Check sheet for the drawn part. Datum: minimum x, y, z corner. Units: mm. A direction names the side the tool comes from. Round coordinates to 2 decimals unless told otherwise and drop trailing zeros. Write each loop counter-clockwise with the first axis right and the second up, starting at its lowest first coordinate (ties: lowest second). Pieces come first, ordered by that corner, then holes. Notation, with made-up numbers: M -33.75,29.5 L -25.75,29.5 A26 cw -25.75,68.5 Z; hole C 55.5,6.5 d8. An arc over 180 degrees is marked long. One line per item, written item: value. Start each with the question number.
1. Depth check by flat-ended pin: P1, Ø8, axis at x = 55, z = 13, coming from the -Y side; P2, Ø6, axis at x = 66, z = 6, coming from the +Y side; P3, Ø3, axis at y = 26, z = 15, coming from the -X side; P4, Ø3, axis at x = 9, y = 5.5, coming from the -Z side. Enter the tip coordinate at first touch or a pass-through.
2. Section check B-B (z = 10.5). Count the separate pieces of the cut face and the enclosed holes in it.
3. Section check D-D (y = 38). Record the boundary of the cut face in (x, z), and give its area (3 significant figures).
4. Section check A-A (y = 17). Record the boundary of the cut face in (x, z) (1 decimal), and give its area (3 significant figures).
5. Access from +Z, -Z, +X, -X, +Y, -Y to the whole of each face (thin tool, end or side, straight path). Record for the marked faces 4, 5 and 6.
6. Scan lines: probe 1 along X at (y, z) = (3.5, 5.5); probe 2 along Z at (x, y) = (81.5, 5.5); probe 3 along X at (y, z) = (27, 5) (1 decimal). Record each from-to range of solid material in increasing order. Write a range as [from, to].
7. Release check for a two-part mould opening along X. For the marked faces 1, 2 and 3 record: pulls with the +X half, pulls with the -X half, needs draft (parallel to the pull), parting line crosses it, or undercut.
8. Section check C-C (z = 15.5). Record the boundary of the cut face in (x, y) (1 decimal).
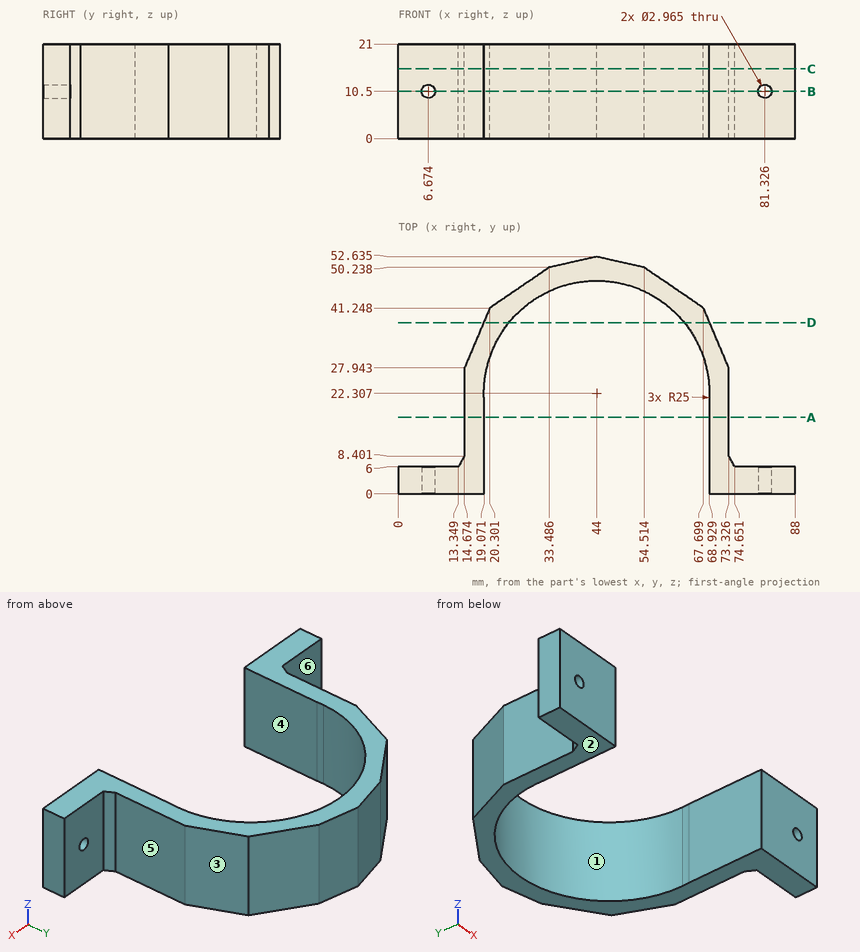
Result sheet:
1. P1: stops at y = 42.31
1. P2: stops at y = 44.45
1. P3: stops at x = 14.67
1. P4: stops at z = 0
2. separate pieces: 3
2. enclosed holes: 0
3. outline: M 18.93,0 L 24.54,0 L 24.54,21 L 18.93,21 Z; M 63.46,0 L 69.07,0 L 69.07,21 L 63.46,21 Z
3. area: 236 mm2
4. outline: M 14.7,0 L 19.1,0 L 19.1,21 L 14.7,21 Z; M 68.9,0 L 73.3,0 L 73.3,21 L 68.9,21 Z
4. area: 185 mm2
5. face 4: +Z, -Z, -Y
5. face 5: +Z, -Z, +X, +Y
5. face 6: +Z, -Z, -X, +Y
6. probe 1: x = [0, 19.07], [68.93, 88]
6. probe 2: z = [0, 9.03], [11.97, 21]
6. probe 3: x = [14.7, 19.4], [68.6, 73.3]
7. face 1: undercut
7. face 2: needs draft
7. face 3: pulls with the +X half
8. outline: M 0,0 L 19.1,0 L 19.1,20.4 A25 cw 19,22.3 A25 cw 69,22.3 A25 cw 68.9,20.4 L 68.9,0 L 88,0 L 88,6 L 74.7,6 L 73.3,8.4 L 73.3,27.9 L 67.7,41.2 L 54.5,50.2 L 44,52.6 L 33.5,50.2 L 20.3,41.2 L 14.7,27.9 L 14.7,8.4 L 13.3,6 L 0,6 Z
